Model file for the job. Use its own axes, mm. Coordinates: 2 decimals unless noted, no trailing zeros. Loops run counter-clockwise (first coordinate to the right, second up) from the corner with the lowest first, then second, coordinate; pieces in that order, holes last.
from build123d import *

# Parameters (mm, degrees)
BOSS_EXTRUDE1_DEPTH       = 5
SKETCH2_R                 = 4.1
BOSS_EXTRUDE2_DEPTH       = 7
F_2_0MM_DOWEL_HOLE2_D     = 2
F_2_0MM_DOWEL_HOLE2_DEPTH = 7
F_2_0MM_DOWEL_HOLE2_TIP   = 0.600860619


with BuildPart() as part:
    # Sketch1 → Boss-Extrude1 (new body)
    with BuildSketch(Plane(origin=(0, 0, 0), x_dir=(1, 0, 0), z_dir=(0, 1, 0))):
        with BuildLine():
            Line((0, 26), (0, 0))
            Line((0, 0), (35, 0))
            ThreePointArc((35, 0), (22, 13), (35, 26))
            Line((35, 26), (0, 26))
        make_face()
        with BuildLine():
            ThreePointArc((35, 26), (22, 13), (35, 0))
            Line((35, 0), (35, 26))
        make_face()
        with BuildLine():
            Line((35, 26), (35, 0))
            ThreePointArc((35, 0), (44.192388155, 3.807611845), (48, 13))
            ThreePointArc((48, 13), (44.192388155, 22.192388155), (35, 26))
        make_face()
    extrude(amount=BOSS_EXTRUDE1_DEPTH)

    # Sketch2 → Boss-Extrude2 (add)
    with BuildSketch(Plane(origin=(0, 5, 0), x_dir=(1, 0, 0), z_dir=(0, 1, 0))):
        with Locations(Location((35, 13, 0), (0, 0, 270))):
            Circle(SKETCH2_R)
    extrude(amount=BOSS_EXTRUDE2_DEPTH)

    # Ø2.0mm Dowel Hole2
    with Locations(Plane.XZ):
        with Locations((2.5, -6.5), (2.5, -12.1), (2.5, -18.6)):
            Hole(F_2_0MM_DOWEL_HOLE2_D / 2, depth=F_2_0MM_DOWEL_HOLE2_DEPTH)
            with Locations((0, 0, -(F_2_0MM_DOWEL_HOLE2_DEPTH + F_2_0MM_DOWEL_HOLE2_TIP / 2))):  # 118° drill point
                Cone(0, F_2_0MM_DOWEL_HOLE2_D / 2, F_2_0MM_DOWEL_HOLE2_TIP, mode=Mode.SUBTRACT)


solid = part.part
Q1. Slice it at C-C (y = 2.25). List the corners of the cut face in (x, z).
Answers:
outline: (0, -26) - (35, -26) arc R13 ccw to (35, 0) - (0, 0) - close; hole circle Ø2 at (2.5, -18.6); hole circle Ø2 at (2.5, -12.1); hole circle Ø2 at (2.5, -6.5)
Q2. Slice it at A-A (x = 2.5). List the corners of the cut face in (y, z).
Answers:
outline: (0, -26) - (5, -26) - (5, -19.6) - (0, -19.6) - close; (0, -17.6) - (5, -17.6) - (5, -13.1) - (0, -13.1) - close; (0, -11.1) - (5, -11.1) - (5, -7.5) - (0, -7.5) - close; (0, -5.5) - (5, -5.5) - (5, 0) - (0, 0) - close
Q3. Mould opens along Z. For faces 1 (the flat face through (0, 2, -13)), 2 (the cylindrical face through (37.771, 8.451, -16.022)), 3 (the cylindrical face through (2.63, 2.54, -11.11)), 4 (the flat face through (18, 2, -26)) say: +Z half, -Z half, draft (parallel to the pull), parting line (faces both ways), or undercut.
Answers:
face 1: draft
face 2: parting line
face 3: undercut
face 4: -Z half
Q4. Flat gauge pins, fed straight in: P1, Ø3, axis at x = 2.5, z = -12.1, coming from the -Y side; P2, Ø2.5, axis at x = 2.5, z = -18.6, coming from the +Y side; P3, Ø5, axis at y = 5.5, z = -22.5, coming from the +X side. Where does each tip first touch, or does it go through?
Answers:
P1: stops at y = 0
P2: stops at y = 5
P3: stops at x = 45.92
Q5. Slice it at D-D (y = 7). List the corners of the cut face in (x, z), and give its area (3 significant figures).
Answers:
outline: circle Ø8.2 at (35, -13)
area: 52.8 mm2
Q6. Slice it at B-B (z = -18.6). List the corners of the cut face in (x, y).
Answers:
outline: (0, 0) - (1.5, 0) - (1.5, 5) - (0, 5) - close; (3.5, 0) - (46.73, 0) - (46.73, 5) - (3.5, 5) - close
Q7. Drill centre lines: line 1 (Z direction, x = 2.5, y = 3.3); line 2 (Y direction, x = 15, z = -11.5); line 3 (X direction, y = 1.5, z = -19.25). Where is each one in solid material? Low to high.
Answers:
line 1: z = -26 to -19.6, -17.6 to -13.1, -11.1 to -7.5, -5.5 to 0
line 2: y = 0 to 5
line 3: x = 0 to 1.74, 3.26 to 46.4
